Part model, mm, in its own coordinate system. A direction names the side the tool comes from. Round coordinates to 2 decimals unless told otherwise and drop trailing zeros. Loops run counter-clockwise (first coordinate to the right, second up) from the corner with the lowest first, then second, coordinate; pieces in that order, holes last. Notation, with made-up numbers: (28, 36.25) -> (77, 36.25) arc R8 ccw to (77, 44.25) -> close; hole circle Ø5 at (3.25, 33.25). An arc over 180 degrees is marked (long way). Use a Markdown table: item, result. Add a question column.
Item 1: Cut at B-B, the plane x = 0. List the corners of the cut face in (y, z), plus the area to 3 significant figures.
Item 2: Cut at D-D, the plane z = -2.25. List the corners of the cut face in (x, y), plus the area to 3 significant figures.
Item 3: Cut at C-C, the plane y = 6.75. List the corners of the cut face in (x, z).
Item 4: Probe line 1 (Y direction, x = 1.25, z = -0.5); line 2 (Z direction, x = 1.5, y = 7); line 3 (Z direction, x = -1, y = 7.75). List the from-to ranges inside material, lowest first. Write a range as [from, to].
Item 5: Cut at A-A, the plane z = 0. List the corners of the cut face in (x, y).
Item 6: Which spindle directions (+Z, -Z, +X, -X, +Y, -Y) get a long thin tool onto all of the face, cutting with end or side? Do faces 4 (the face through (0, 0, 0)), 5 (the face through (2, 10, 2)), 6 (the face through (0, 11.8, 0)). Say none if no direction does.
Item 7: Flat gauge pins, fed straight in: pin 1 (1.6 mm diameter, centred on x = 0.5, y = 13, fed in from -Z); pin 2 (1.6 mm diameter, centred on x = -2, y = 12, fed in from +Z); pin 3 (1.5 mm diameter, centred on x = 1.5, z = 3, fed in from -Y); pin 4 (2 mm diameter, centred on y = 4.5, z = 0.5, fed in from +X). Where does each tip first touch, or does it go through?
Item 8: Two-plate mould, pull along Z, no slides. Class faces 1 (the face through (0, 13.3, -2)), 2 (the face through (3.77, 11.67, -1.96)), 3 (the face through (0, 13, 0.63)): pulls with the +Z half, pulls with the -Z half, needs draft (parallel to the pull), parting line crosses it, or undercut.
```python
from build123d import *

# Parameters (mm, degrees)
CUT_EXTRUDE_1_DEPTH = 1.5


with BuildPart() as part:
    # Эскиз1 → Revolve 256 (revolve)
    with BuildSketch(Plane.XY, mode=Mode.PRIVATE) as revolve_256_sk:
        Polygon((0, 0), (2.5, 0), (2.5, 10), (4.25, 10), (4.25, 13.3), (0, 13.3), align=None)
    revolve(revolve_256_sk.sketch.rotate(Axis((0, 0, 0), (0, 1, 0)), 90), axis=Axis((0, 0, 0), (0, 1, 0)))

    # Эскиз2 → Вырез-Вытянуть1 (cut)
    with BuildSketch(Plane(origin=(0, 13.3, 0), x_dir=(-1, 0, 0), z_dir=(0, 1, 0))):
        with BuildLine():
            Line((-4.203046514, -0.63), (4.203046514, -0.63))
            ThreePointArc((4.203046514, -0.63), (4.25, 0), (4.203046514, 0.63))
            Line((4.203046514, 0.63), (-4.203046514, 0.63))
            ThreePointArc((-4.203046514, 0.63), (-4.25, 0), (-4.203046514, -0.63))
        make_face()
    extrude(amount=-CUT_EXTRUDE_1_DEPTH, mode=Mode.SUBTRACT)


solid = part.part
```
A:
| question | item | result |
|---|---|---|
| 1 | outline | (0, -2.5) -> (10, -2.5) -> (10, -4.25) -> (13.3, -4.25) -> (13.3, -0.63) -> (11.8, -0.63) -> (11.8, 0.63) -> (13.3, 0.63) -> (13.3, 4.25) -> (10, 4.25) -> (10, 2.5) -> (0, 2.5) -> close |
| 1 | area | 76.2 mm^2 |
| 2 | outline | (-3.61, 10) -> (-1.09, 10) -> (-1.09, 0) -> (1.09, 0) -> (1.09, 10) -> (3.61, 10) -> (3.61, 13.3) -> (-3.61, 13.3) -> close |
| 2 | area | 45.6 mm^2 |
| 3 | outline | circle Ø5 at (0, 0) |
| 4 | line 1 | y = [0, 11.8] |
| 4 | line 2 | z = [-2, 2] |
| 4 | line 3 | z = [-2.29, 2.29] |
| 5 | outline | (-4.25, 10) -> (-2.5, 10) -> (-2.5, 0) -> (2.5, 0) -> (2.5, 10) -> (4.25, 10) -> (4.25, 11.8) -> (-4.25, 11.8) -> close |
| 6 | face 4 | +Z, -Z, +X, -X, -Y |
| 6 | face 5 | -Y |
| 6 | face 6 | +X, -X, +Y |
| 7 | pin 1 | stops at z = -4.25 |
| 7 | pin 2 | stops at z = 4.08 |
| 7 | pin 3 | stops at y = 10 |
| 7 | pin 4 | stops at x = 2.5 |
| 8 | face 1 | needs draft |
| 8 | face 2 | parting line crosses it |
| 8 | face 3 | undercut |
